Design review of the part built by this model. Coordinates are the model's own, in mm. A direction names the side the tool comes from. Coordinates: 2 decimals unless noted, no trailing zeros. Loops run counter-clockwise (first coordinate to the right, second up) from the corner with the lowest first, then second, coordinate; pieces in that order, holes last. Notation, with made-up numbers: (22.25, 2) -> (62.25, 2) arc R30 ccw to (62.25, 34) -> close; hole circle Ø4 at (7, 11.5). An arc over 180 degrees is marked (long way). Use CSV: the item, a comma, the result in double quotes.
```python
from build123d import *

# Parameters (mm, degrees)
F0_W     = 381
F0_H     = 304.8
F1_DEPTH = 19.05
F3_DEPTH = 457.2
F4_W     = 307.975
F4_H     = 431.8
F5_DEPTH = 6.35
F6_W     = 307.975
F6_H     = 431.8
F7_DEPTH = 247.65


with BuildPart() as f1:
    # F0 (on Front) → F1 (new body)
    with BuildSketch(Plane.XZ):
        Rectangle(F0_W, F0_H)
    extrude(amount=F1_DEPTH)

    # F2 (on face) → F3 (join)
    with BuildSketch(Plane(origin=(0, 0, 0), x_dir=(-1, 0, 0), z_dir=(0, 1, 0))):
        Polygon((-166.6875, -130.175), (0, -130.175), (166.6875, -130.175), (166.6875, 130.175), (-166.6875, 130.175), align=None)
    extrude(amount=F3_DEPTH)

    # F4 (on face) → F5 (cut)
    with BuildSketch(Plane(origin=(0, 0, -130.175), x_dir=(1, 0, 0), z_dir=(0, 0, -1))):
        with Locations((0, -228.6)):
            Rectangle(F4_W, F4_H)
    extrude(amount=-F5_DEPTH, mode=Mode.SUBTRACT)

    # F6 (on face) → F7 (cut)
    with BuildSketch(Plane.XY.offset(130.175)):
        with Locations((0, 228.6)):
            Rectangle(F6_W, F6_H)
    extrude(amount=-F7_DEPTH, mode=Mode.SUBTRACT)


solid = f1.part
```
Item 1: Add section B-B (y = 171). Give the boundary of the cut face in (x, z) (1 decimal), then the cut area to 3 significant figures.
Checked values:
outline,"(-166.7, -130.2) -> (-154, -130.2) -> (-154, -123.8) -> (154, -123.8) -> (154, -130.2) -> (166.7, -130.2) -> (166.7, 130.2) -> (154, 130.2) -> (154, -117.5) -> (-154, -117.5) -> (-154, 130.2) -> (-166.7, 130.2) -> close"
area,"8,570 mm^2"
Item 2: Machinability: for faces 1 (the face through (-161, 228, 130.175)), 2 (the face through (161, 228, -130.175)), 3 (the face through (153.988, 226, 8)), 4 (the face through (166.688, 225, 2)), which of the approach directions +Z, -Z, +X, -X, +Y, -Y give a long, thin tool a straight path to every point of the face, cutting with its end or side? Answer none if there is none.
Checked values:
face 1,"+Z, +X, -X, +Y"
face 2,"-Z, +X, -X, +Y"
face 3,"+Z"
face 4,"+Z, -Z, +X, +Y"
Item 3: Add section C-C (x = 143.5). Give the boundary of the cut face in (y, z) (3 decimals).
Checked values:
outline,"(-19.05, -152.4) -> (0, -152.4) -> (0, -130.175) -> (12.7, -130.175) -> (12.7, -123.825) -> (444.5, -123.825) -> (444.5, -130.175) -> (457.2, -130.175) -> (457.2, 130.175) -> (444.5, 130.175) -> (444.5, -117.475) -> (12.7, -117.475) -> (12.7, 130.175) -> (0, 130.175) -> (0, 152.4) -> (-19.05, 152.4) -> close"
Item 4: Add section A-A (z = 45). Give the boundary of the cut face in (x, y).
Checked values:
outline,"(-190.5, -19.05) -> (190.5, -19.05) -> (190.5, 0) -> (166.69, 0) -> (166.69, 457.2) -> (-166.69, 457.2) -> (-166.69, 0) -> (-190.5, 0) -> close; hole (-153.99, 12.7) -> (153.99, 12.7) -> (153.99, 444.5) -> (-153.99, 444.5) -> close"
Item 5: Clearance check with flat-ended pins moving along their axes: pin 1 (2 mm diameter, centred on x = 91, y = 383.5, fed in from +Z) (3 decimals); pin 2 (1 mm diameter, centred on y = 385.5, z = -55, fed in from -X); pin 3 (5 mm diameter, centred on y = 341, z = 44, fed in from +X). State where each tip first meets the part, or that it passes through.
Checked values:
pin 1,"z = -117.475"
pin 2,"x = -166.69"
pin 3,"x = 166.69"
Item 6: To check wall thickness, follow line 1 along Y through (x, z) = (-150.5, -30); line 2 along X through (y, z) = (366, -107.5); line 3 along Z through (x, y) = (-82, 341) (3 decimals). State the ranges of each line that lie inside material, in increasing order.
Checked values:
line 1,"-19.05 to 12.7, 444.5 to 457.2"
line 2,"-166.69 to -153.99, 153.99 to 166.69"
line 3,"-123.825 to -117.475"
Item 7: Draft analysis for pull direction X (two halves, no side actions). For faces 5 (the face through (-166.688, 225, -2)), 6 (the face through (190.5, -9, -2)), 7 (the face through (-2, 226, -123.825)), 8 (the face through (-153.988, 226, 8)), state which applies: pulls with the +X half, pulls with the -X half, needs draft (parallel to the pull), parting line crosses it, or undercut.
Checked values:
face 5,"pulls with the -X half"
face 6,"pulls with the +X half"
face 7,"undercut"
face 8,"undercut"
